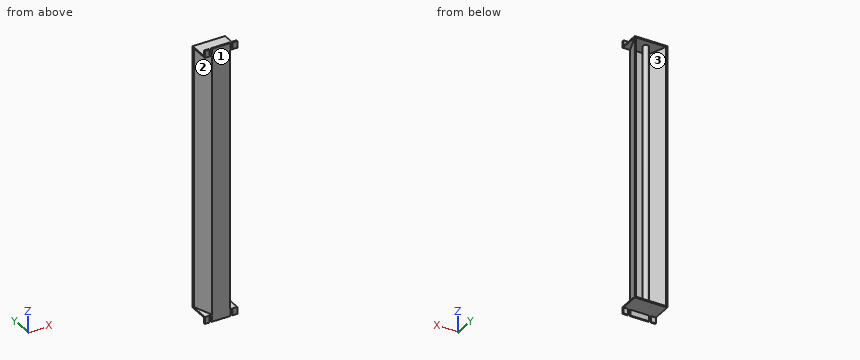
from build123d import *

# Parameters (mm, degrees)
SKETCH_1_W             = 56
SKETCH_1_H             = 35
EXTRUDE_1_DEPTH        = 2
EXTRUDE_2_DEPTH        = 225
EXTRUDE_START          = -12
EXTRUDE_5_DEPTH        = 10
SKETCH_16_R            = 5
EXTRUDE_6_DEPTH        = 225
SKETCH_15_W            = 4
SKETCH_15_H            = 10
CUT_EXTRUDE_1_DEPTH    = 10
MIRROR_START           = 225
MIRROR_1_OUTLINE_R     = 5
MIRROR_1_DEPTH         = 227
MIRROR_START_2         = 450
MIRROR_1_2_OUTLINE_R   = 5
MIRROR_1_2_DEPTH       = 2
MIRROR_START_3         = 452
MIRROR_1_3_OUTLINE_W   = 32
MIRROR_1_3_OUTLINE_H   = 2
MIRROR_1_3_OUTLINE_W_2 = 8
MIRROR_1_3_DEPTH       = 10


# Read off the part's stored shape, not the designer's step: 凸台-拉伸2, 镜向1
with BuildPart() as part:
    # 草图1 (on Front Plane) → 凸台-拉伸1 (new body)
    with BuildSketch(Plane.XY):
        with Locations((28, 17.5)):
            Rectangle(SKETCH_1_W, SKETCH_1_H)
    extrude(amount=-EXTRUDE_1_DEPTH)

    # 凸台-拉伸2 outline → 凸台-拉伸2 (add)
    with BuildSketch(Plane.XY):
        Polygon((0, 35), (0, 33), (0.727940469, 33), (12.738958199, 0), (43.261041801, 0), (55.272059531, 33), (56, 33), (56, 35), (53.871644455, 35), (41.860626724, 2), (14.139373276, 2), (2.128355545, 35), align=None)
    extrude(amount=EXTRUDE_2_DEPTH)

    # 草图1<10> (on Front Plane) → 凸台-拉伸5 (add)
    with BuildSketch(Plane.XY.offset(EXTRUDE_START)):
        Polygon((28, 2), (14.139373276, 2), (14.867313744, 0), (28, 0), align=None)
        Polygon((14.139373276, 2), (12.011017731, 2), (12.738958199, 0), (14.867313744, 0), align=None)
        Polygon((12.738958199, 0), (12.011017731, 2), (0, 2), (0, 0), align=None)
        Polygon((41.860626724, 2), (28, 2), (28, 0), (41.132686256, 0), align=None)
        Polygon((56, 2), (43.988982269, 2), (43.261041801, 0), (56, 0), align=None)
        Polygon((43.988982269, 2), (41.860626724, 2), (41.132686256, 0), (43.261041801, 0), align=None)
    extrude(amount=EXTRUDE_5_DEPTH)

    # 草图16 → 凸台-拉伸6 (add)
    with BuildSketch(Plane.XY):
        with Locations((28, 20)):
            Circle(SKETCH_16_R)
    extrude(amount=EXTRUDE_6_DEPTH)

    # 草图15 → 切除-拉伸1 (cut)
    with BuildSketch(Plane(origin=(0, 2, 0), x_dir=(1, 0, 0), z_dir=(0, 1, 0))):
        with Locations((46, -457)):
            Rectangle(SKETCH_15_W, SKETCH_15_H)
        with Locations((10, 7)):
            Rectangle(SKETCH_15_W, SKETCH_15_H)
        with Locations((46, 7)):
            Rectangle(SKETCH_15_W, SKETCH_15_H)
        with Locations((10, -457)):
            Rectangle(SKETCH_15_W, SKETCH_15_H)
    extrude(amount=-CUT_EXTRUDE_1_DEPTH, mode=Mode.SUBTRACT)

    # 镜向1 outline → 镜向1 (add)
    with BuildSketch(Plane.XY.offset(MIRROR_START)):
        Polygon((43.261041801, 0), (55.272059531, 33), (56, 33), (56, 35), (53.871644455, 35), (41.860626724, 2), (14.139373276, 2), (2.128355545, 35), (0, 35), (0, 33), (0.727940469, 33), (12.738958199, 0), align=None)
        with Locations((28, 20)):
            Circle(MIRROR_1_OUTLINE_R)
    extrude(amount=MIRROR_1_DEPTH)

    # Mirror 1 2 outline → Mirror 1 2 (add)
    # profile 1 of 3: a face of its own
    with BuildSketch(Plane.XY.offset(MIRROR_START_2)):
        Polygon((14.139373276, 2), (41.860626724, 2), (53.871644455, 35), (2.128355545, 35), align=None)
        with Locations((28, 20)):
            Circle(MIRROR_1_2_OUTLINE_R, mode=Mode.SUBTRACT)
    # profile 2 of 3: a face of its own
    with BuildSketch(Plane.XY.offset(MIRROR_START_2)):
        Polygon((55.272059531, 33), (43.261041801, 0), (56, 0), (56, 33), align=None)
    # profile 3 of 3: a face of its own
    with BuildSketch(Plane.XY.offset(MIRROR_START_2)):
        Polygon((12.738958199, 0), (0.727940469, 33), (0, 33), (0, 0), align=None)
    extrude(amount=MIRROR_1_2_DEPTH)

    # Mirror 1 3 outline → Mirror 1 3 (add)
    with BuildSketch(Plane.XY.offset(MIRROR_START_3)):
        with Locations((28, 1)):
            Rectangle(MIRROR_1_3_OUTLINE_W, MIRROR_1_3_OUTLINE_H)
        with Locations((52, 1)):
            Rectangle(MIRROR_1_3_OUTLINE_W_2, MIRROR_1_3_OUTLINE_H)
        with Locations((4, 1)):
            Rectangle(MIRROR_1_3_OUTLINE_W_2, MIRROR_1_3_OUTLINE_H)
    extrude(amount=MIRROR_1_3_DEPTH)


solid = part.part
The listing builds one solid part. Answer for the finished solid, in the listing's coordinates (mm). Face numbers are marked on the shaded views. Give positions to 0.01 mm unless a question says otherwise; leave off trailing zeros. Loops run counter-clockwise (first coordinate to the right, second up) from the corner with the lowest first, then second, coordinate; pieces in that order, holes last.
Item 1: Determine the mould class of the marked faces 1, 2 and 3 for opening direction X: +X half, -X half, draft (parallel to the pull), parting line (faces both ways), or undercut.
Derived:
face 1: draft
face 2: -X half
face 3: undercut
Item 2: Each of these flat-tipped pins is pushed along its axis until it touches: pin 1 Ø6.5 at (x, z) = (5.5, 459) entering from +Y; pin 2 Ø1.5 at (y, z) = (26, 195.5) entering from +X; pin 3 Ø4 at (x, y) = (48, 24.5) entering from -Z. Where does it stop, or does it pass through?
Derived:
pin 1: stops at y = 2
pin 2: stops at x = 53
pin 3: stops at z = -2
Item 3: A cutting plane is placed at A-A (z = 280). Give the vertices of the cut face in (x, y), then the cut area to 3 significant figures.
Derived:
outline: (0, 33) - (0.73, 33) - (12.74, 0) - (43.26, 0) - (55.27, 33) - (56, 33) - (56, 35) - (53.87, 35) - (41.86, 2) - (14.14, 2) - (2.13, 35) - (0, 35) - close; circle Ø10 at (28, 20)
area: 283 mm2
Item 4: A cutting plane is placed at C-C (y = 20). Give the vertices of the cut face in (x, z).
Derived:
outline: (0, -2) - (56, -2) - (56, 0) - (50.54, 0) - (50.54, 450) - (56, 450) - (56, 452) - (0, 452) - (0, 450) - (5.46, 450) - (5.46, 0) - (0, 0) - close; hole (7.59, 0) - (23, 0) - (23, 450) - (7.59, 450) - close; hole (33, 0) - (48.41, 0) - (48.41, 450) - (33, 450) - close
Item 5: A cutting plane is placed at B-B (x = 28). Give the vertices of the cut face in (y, z).
Derived:
outline: (0, -12) - (2, -12) - (2, -2) - (35, -2) - (35, 0) - (25, 0) - (25, 450) - (35, 450) - (35, 452) - (2, 452) - (2, 462) - (0, 462) - close; hole (2, 0) - (15, 0) - (15, 450) - (2, 450) - close
Item 6: Find the intervals of material crossed by line 1 along Z through (x, y) = (52, 3.5); line 2 along X through (y, z) = (17.5, 316.5); line 3 along Y through (x, z) = (17, 15.5), in increasing order.
Derived:
line 1: z = -2 to 0, 450 to 452
line 2: x = 6.37 to 8.5, 23.67 to 32.33, 47.5 to 49.63
line 3: y = 0 to 2
